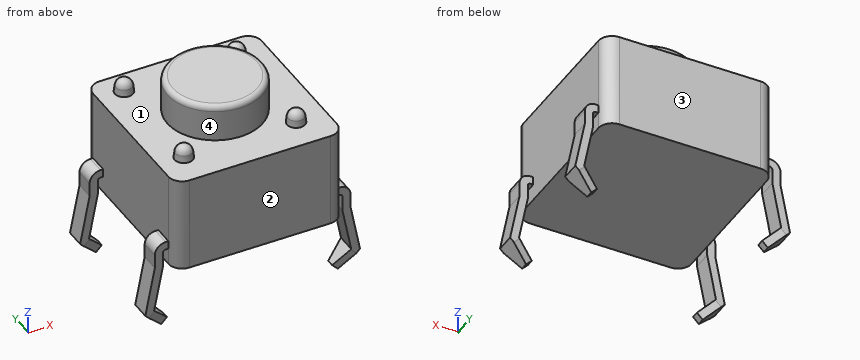
```python
from build123d import *
from OCP.BRepFilletAPI import BRepFilletAPI_MakeChamfer

# Parameters (mm, degrees)
SKETCH1_W                 = 6.2
SKETCH1_H                 = 6.2
EXTRUDE1_DEPTH            = 3.5
SKETCH2_R                 = 1.75
EXTRUDE2_DEPTH            = 1.35
LPATTERN1_COUNT           = 2
LPATTERN1_PITCH           = 4.13
LPATTERN1_COUNT_DIR2      = 2
LPATTERN1_PITCH_DIR2      = 4.13
FILLET1_R                 = 0.5
FILLET2_R                 = 0.2
EXTRUDE3_DEPTH            = 0.35
CHAMFER1_SIZE             = 0.8
CHAMFER1_SIZE2            = 0.214359354
CHAMFER1_OF_MIRROR1_SIZE  = 0.8
CHAMFER1_OF_MIRROR1_SIZE2 = 0.214359354
MIRROR2_START             = -2.6
MIRROR2_DEPTH             = 0.7
MIRROR2_START_2           = 1.9
MIRROR2_2_DEPTH           = 0.7
MIRROR2_START_3           = 3.765863992
MIRROR2_3_DEPTH           = 0.3


with BuildPart() as part:
    # Sketch1 → Extrude1 (new body)
    with BuildSketch(Plane.XY):
        Rectangle(SKETCH1_W, SKETCH1_H)
    extrude(amount=EXTRUDE1_DEPTH)

    # Sketch2 → Extrude2 (add)
    with BuildSketch(Plane.XY.offset(3.5)):
        with Locations(Location((0, 0, 0), (0, 0, 180))):
            Circle(SKETCH2_R)
    extrude(amount=EXTRUDE2_DEPTH)

    # Sketch4 → Revolve1 (revolve)
    with BuildSketch(Plane(origin=(0, 2.25, 0), x_dir=(-1, 0, 0), z_dir=(0, 1, 0)), mode=Mode.PRIVATE) as revolve1_sk:
        with BuildLine():
            Line((1.815270458, 3.5), (2.15, 3.5))
            Line((2.15, 3.5), (2.15, 4))
            ThreePointArc((2.15, 4), (1.948488877, 3.937944347), (1.846391659, 3.753461841))
            Line((1.846391659, 3.753461841), (1.815270458, 3.5))
        make_face()
    revolve1 = revolve(revolve1_sk.sketch.rotate(Axis((-2.15, 2.25, 2.844368125), (0, 0, 1)), 180), axis=Axis((-2.15, 2.25, 2.844368125), (0, 0, 1)))

    # LPattern1: Revolve1 2 × 2
    with Locations(*[(i * LPATTERN1_PITCH, -j * LPATTERN1_PITCH_DIR2, 0) for i in range(LPATTERN1_COUNT) for j in range(LPATTERN1_COUNT_DIR2) if (i, j) != (0, 0)]):
        add(revolve1)

    # Fillet1
    fillet1_edges = [part.edges().sort_by_distance(p)[0] for p in [
        (-3.1, 3.1, 1.75),
        (3.1, 3.1, 1.75),
        (3.1, -3.1, 1.75),
        (-3.1, -3.1, 1.75),
    ]]
    fillet(fillet1_edges, radius=FILLET1_R)

    # Fillet2
    fillet2_edges = [part.edges().sort_by_distance(p)[0] for p in [
        (1.75, 0, 4.85),
    ]]
    fillet(fillet2_edges, radius=FILLET2_R)

    # Sketch5 → Extrude3 (add, symmetric)
    with BuildSketch(Plane(origin=(0, 2.25, 0), x_dir=(-1, 0, 0), z_dir=(0, 1, 0))):
        with BuildLine():
            Line((3.1, 0.91088803), (3.2, 0.91088803))
            ThreePointArc((3.2, 0.91088803), (3.482842712, 0.793730742), (3.6, 0.51088803))
            Line((3.6, 0.51088803), (3.6, 0))
            Line((3.6, 0), (3.95, -1.8))
            Line((3.95, -1.8), (3.25, -2.5))
            Line((3.25, -2.5), (3.037867966, -2.287867966))
            Line((3.037867966, -2.287867966), (3.625066954, -1.700668977))
            Line((3.625066954, -1.700668977), (3.3, -0.02889607))
            Line((3.3, -0.02889607), (3.3, 0.51088803))
            ThreePointArc((3.3, 0.51088803), (3.270710678, 0.581598708), (3.2, 0.61088803))
            Line((3.2, 0.61088803), (3.1, 0.61088803))
            Line((3.1, 0.61088803), (3.1, 0.91088803))
        make_face()
    extrude3 = extrude(amount=EXTRUDE3_DEPTH, both=True)

    # Chamfer1: one chamfer whose edges measure the first distance from different faces: ONE call of the kernel's chamfer builder (chamfer() names one face for all edges)
    chamfer1_edges_1 = [part.edges().sort_by_distance(p)[0] for p in [
        (-3.143933983, 1.9, -2.393933983),
    ]]
    chamfer1_side_1 = [part.faces().sort_by_distance(p)[0] for p in [
        (-3.520562137, 1.9, -0.80393009),
    ]]
    chamfer1_edges_2 = [part.edges().sort_by_distance(p)[0] for p in [
        (-3.143933983, 2.6, -2.393933983),
    ]]
    chamfer1_side_2 = [part.faces().sort_by_distance(p)[0] for p in [
        (-3.520562137, 2.6, -0.80393009),
    ]]
    chamfer1 = BRepFilletAPI_MakeChamfer(part.part.solid().wrapped)
    for e in chamfer1_edges_1:
        chamfer1.Add(CHAMFER1_SIZE, CHAMFER1_SIZE2, e.wrapped, chamfer1_side_1[0].wrapped)  # the first distance lies on this face
    for e in chamfer1_edges_2:
        chamfer1.Add(CHAMFER1_SIZE, CHAMFER1_SIZE2, e.wrapped, chamfer1_side_2[0].wrapped)  # the first distance lies on this face
    add(Compound.cast(chamfer1.Shape()), mode=Mode.REPLACE)

    # Mirror1: Extrude3 across plane
    add(extrude3.mirror(Plane.ZX))

    # Chamfer1 of Mirror1: one chamfer whose edges measure the first distance from different faces: ONE call of the kernel's chamfer builder (chamfer() names one face for all edges)
    chamfer1_of_mirror1_edges_1 = [part.edges().sort_by_distance(p)[0] for p in [
        (-3.143933983, -1.9, -2.393933983),
    ]]
    chamfer1_of_mirror1_side_1 = [part.faces().sort_by_distance(p)[0] for p in [
        (-3.520562137, -1.9, -0.80393009),
    ]]
    chamfer1_of_mirror1_edges_2 = [part.edges().sort_by_distance(p)[0] for p in [
        (-3.143933983, -2.6, -2.393933983),
    ]]
    chamfer1_of_mirror1_side_2 = [part.faces().sort_by_distance(p)[0] for p in [
        (-3.520562137, -2.6, -0.80393009),
    ]]
    chamfer1_of_mirror1 = BRepFilletAPI_MakeChamfer(part.part.solid().wrapped)
    for e in chamfer1_of_mirror1_edges_1:
        chamfer1_of_mirror1.Add(CHAMFER1_OF_MIRROR1_SIZE, CHAMFER1_OF_MIRROR1_SIZE2, e.wrapped, chamfer1_of_mirror1_side_1[0].wrapped)  # the first distance lies on this face
    for e in chamfer1_of_mirror1_edges_2:
        chamfer1_of_mirror1.Add(CHAMFER1_OF_MIRROR1_SIZE, CHAMFER1_OF_MIRROR1_SIZE2, e.wrapped, chamfer1_of_mirror1_side_2[0].wrapped)  # the first distance lies on this face
    add(Compound.cast(chamfer1_of_mirror1.Shape()), mode=Mode.REPLACE)

    # Mirror2: read off the stored shape, not the designer's step
    # Mirror2 outline → Mirror2 (add)
    with BuildSketch(Plane(origin=(0, 0, 0), x_dir=(1, 0, 0), z_dir=(0, 1, 0)).offset(MIRROR2_START)):
        with BuildLine():
            ThreePointArc((3.3, -0.51088803), (3.270710678, -0.581598708), (3.2, -0.61088803))
            Line((3.2, -0.61088803), (3.1, -0.61088803))
            Line((3.1, -0.61088803), (3.1, -0.91088803))
            Line((3.1, -0.91088803), (3.2, -0.91088803))
            ThreePointArc((3.2, -0.91088803), (3.482842712, -0.793730742), (3.6, -0.51088803))
            Line((3.6, -0.51088803), (3.6, 0))
            Line((3.6, 0), (3.95, 1.8))
            Line((3.95, 1.8), (3.25, 2.5))
            Line((3.25, 2.5), (3.037867966, 2.287867966))
            Line((3.037867966, 2.287867966), (3.625066954, 1.700668977))
            Line((3.625066954, 1.700668977), (3.3, 0.02889607))
            Line((3.3, 0.02889607), (3.3, -0.51088803))
        make_face()
    extrude(amount=MIRROR2_DEPTH)

    # Mirror2 2 outline → Mirror2 2 (add)
    with BuildSketch(Plane(origin=(0, 0, 0), x_dir=(1, 0, 0), z_dir=(0, 1, 0)).offset(MIRROR2_START_2)):
        with BuildLine():
            ThreePointArc((3.3, -0.51088803), (3.270710678, -0.581598708), (3.2, -0.61088803))
            Line((3.2, -0.61088803), (3.1, -0.61088803))
            Line((3.1, -0.61088803), (3.1, -0.91088803))
            Line((3.1, -0.91088803), (3.2, -0.91088803))
            ThreePointArc((3.2, -0.91088803), (3.482842712, -0.793730742), (3.6, -0.51088803))
            Line((3.6, -0.51088803), (3.6, 0))
            Line((3.6, 0), (3.95, 1.8))
            Line((3.95, 1.8), (3.25, 2.5))
            Line((3.25, 2.5), (3.037867966, 2.287867966))
            Line((3.037867966, 2.287867966), (3.625066954, 1.700668977))
            Line((3.625066954, 1.700668977), (3.3, 0.02889607))
            Line((3.3, 0.02889607), (3.3, -0.51088803))
        make_face()
    extrude(amount=MIRROR2_2_DEPTH)

    # Mirror2 3 outline → Mirror2 3 (cut)
    with BuildSketch(Plane(origin=(0, 0, 0), x_dir=(0.7071067811865487, 0, 0.7071067811865464), z_dir=(0.7071067811865465, 0, -0.7071067811865485)).offset(MIRROR2_START_3)):
        Polygon((0.530330086, -2.6), (1.330330086, -2.6), (0.530330086, -2.385640646), align=None)
        Polygon((0.530330086, -1.9), (0.530330086, -2.114359354), (1.330330086, -1.9), align=None)
        Polygon((1.330330086, 1.9), (0.530330086, 2.114359354), (0.530330086, 1.9), align=None)
        Polygon((0.530330086, 2.385640646), (1.330330086, 2.6), (0.530330086, 2.6), align=None)
    extrude(amount=MIRROR2_3_DEPTH, mode=Mode.SUBTRACT)


solid = part.part
```
For this review, take the finished solid that the model builds, in its own axes (mm). Face numbers are marked on the shaded views. A direction names the side the tool comes from. Give positions to 0.01 mm unless a question says otherwise; leave off trailing zeros. Write each loop counter-clockwise with the first axis right and the second up, starting at its lowest first coordinate (ties: lowest second). Pieces come first, ordered by that corner, then holes.
Item 1: Take a section at B-B (z = 3). Give the boundary of the cut face in (x, y), and give its area (3 significant figures).
Item 2: Machinability: for the marked faces 3 and 4, which of the approach directions +Z, -Z, +X, -X, +Y, -Y give a long, thin tool a straight path to every point of the face, cutting with its end or side? Answer none if there is none.
Item 3: Insertion check: P1, Ø1, axis at y = -0.5, z = 3, coming from the +X side; P2, Ø3, axis at y = -2, z = 4, coming from the -X side. Each pin has a flat end and moves straight along its axis. Give the tip position at first contact, or say it passes through.
Item 4: Take a section at A-A (y = 0). Give the boundary of the cut face in (x, z).
Item 5: Take a section at D-D (z = 4.25). Give the boundary of the cut face in (x, y), and give its area (3 significant figures).
Item 6: The part is to be moulded in two halves that separate along X. For the marked faces 1 and 2, say which applies: +X half, -X half, draft (parallel to the pull), parting line (faces both ways), or undercut.
Item 7: Wall thickness on probe 1 along Z at (x, y) = (-2, 1.75); probe 2 along X at (y, z) = (-1.25, 0.25); probe 3 along X at (y, z) = (2.25, -0.75): over which ranges is each line inside the solid? List them lowest first.
Established:
1. outline: (-3.1, -2.6) arc R0.5 ccw to (-2.6, -3.1) - (2.6, -3.1) arc R0.5 ccw to (3.1, -2.6) - (3.1, 2.6) arc R0.5 ccw to (2.6, 3.1) - (-2.6, 3.1) arc R0.5 ccw to (-3.1, 2.6) - close
1. area: 38.2 mm2
2. face 3: +Z, -Z, +X, -X, +Y
2. face 4: +Z
3. P1: stops at x = 3.1
3. P2: stops at x = -3.1
4. outline: (-3.1, 0) - (3.1, 0) - (3.1, 3.5) - (1.75, 3.5) - (1.75, 4.65) arc R0.2 ccw to (1.55, 4.85) - (-1.55, 4.85) arc R0.2 ccw to (-1.75, 4.65) - (-1.75, 3.5) - (-3.1, 3.5) - close
5. outline: circle Ø3.5 at (0, 0)
5. area: 9.62 mm2
6. face 1: undercut
6. face 2: draft
7. probe 1: z = 0 to 3.5
7. probe 2: x = -3.1 to 3.1
7. probe 3: x = -3.75 to -3.44, 3.44 to 3.75
